The listing builds one solid part. Answer for the finished solid, in the listing's coordinates (mm). Face numbers are marked on the shaded views. A direction names the side the tool comes from. Give positions to 0.01 mm unless a question says otherwise; leave off trailing zeros. Order: outer loops, then holes, each group sorted by start corner. A loop starts at its lowest first (then second) coordinate and runs counter-clockwise, first axis right, second up. Notation, with made-up numbers: (85, -30) - (114, -30) arc R22 cw to (114, -7) - close; hole circle Ø9 at (41.5, 36). An arc over 180 degrees is marked (long way). Answer in a Markdown table with one row per item.
from build123d import *

# Parameters (mm, degrees)
F0_W     = 20
F0_H     = 20
F0_W_2   = 5
F0_H_2   = 10
F0_R     = 2.5
F1_DEPTH = 2


with BuildPart() as f1:
    # F0 (on Top) → F1 (new body)
    with BuildSketch(Plane.XY):
        Rectangle(F0_W, F0_H)
        with Locations((-5, 0)):
            Rectangle(F0_W_2, F0_H_2, mode=Mode.SUBTRACT)
        with Locations((5, 0)):
            Circle(F0_R, mode=Mode.SUBTRACT)
    extrude(amount=F1_DEPTH)


solid = f1.part
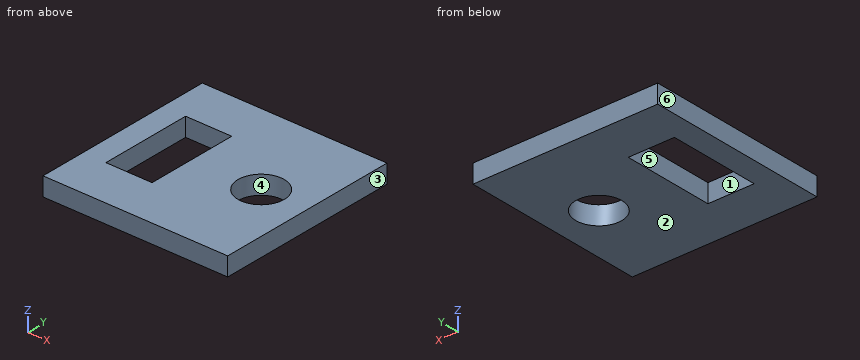
Item 1: Determine the mould class of the marked faces 3, 4, 5 and 6 for opening direction X: pulls with the +X half, pulls with the -X half, needs draft (parallel to the pull), parting line crosses it, or undercut.
Answer block:
| item | result |
|---|---|
| face 3 | pulls with the +X half |
| face 4 | undercut |
| face 5 | undercut |
| face 6 | pulls with the -X half |
Item 2: Consider line 1 (X direction, y = 2.75, z = 0.2); line 2 (Y direction, x = -7, z = 1.5); line 3 (Y direction, x = 5, z = 1.45). Determine where each line is inside the solid, lowest interval first.
Answer block:
| item | result |
|---|---|
| line 1 | -10 to -7.5, -2.5 to 10 |
| line 2 | -10 to -5, 5 to 10 |
| line 3 | -10 to -2.5, 2.5 to 10 |
Item 3: Which of the six approach directions +Z, -Z, +X, -X, +Y, -Y give full straight-line access (tool end or side, diameter ignored) to the marked faces 1 and 2?
Answer block:
| item | result |
|---|---|
| face 1 | +Z, -Z |
| face 2 | -Z, +X, -X, +Y, -Y |
Item 4: Find section B-B on z = 1.7. Write down the section's boundary in (x, y).
Answer block:
| item | result |
|---|---|
| outline | (-10, -10) - (10, -10) - (10, 10) - (-10, 10) - close; hole (-7.5, -5) - (-2.5, -5) - (-2.5, 5) - (-7.5, 5) - close; hole circle Ø5 at (5, 0) |
Item 5: Find section D-D on x = 5. Write down the section's boundary in (y, z).
Answer block:
| item | result |
|---|---|
| outline | (-10, 0) - (-2.5, 0) - (-2.5, 2) - (-10, 2) - close; (2.5, 0) - (10, 0) - (10, 2) - (2.5, 2) - close |
Item 6: Find section C-C on y = 0. Write down the section's boundary in (x, z), then the cut area to 3 significant figures.
Answer block:
| item | result |
|---|---|
| outline | (-10, 0) - (-7.5, 0) - (-7.5, 2) - (-10, 2) - close; (-2.5, 0) - (2.5, 0) - (2.5, 2) - (-2.5, 2) - close; (7.5, 0) - (10, 0) - (10, 2) - (7.5, 2) - close |
| area | 20.0 mm² |
Item 7: Find section A-A on x = -3.75. Write down the section's boundary in (y, z), then the cut area to 3 significant figures.
Answer block:
| item | result |
|---|---|
| outline | (-10, 0) - (-5, 0) - (-5, 2) - (-10, 2) - close; (5, 0) - (10, 0) - (10, 2) - (5, 2) - close |
| area | 20.0 mm² |
